Work out the finished part from the listing and answer in its coordinate system (mm). Face numbers are marked on the shaded views. A direction names the side the tool comes from. Coordinates: 2 decimals unless noted, no trailing zeros. Loops run counter-clockwise (first coordinate to the right, second up) from the corner with the lowest first, then second, coordinate; pieces in that order, holes last. Notation, with made-up numbers: (30.25, 65) - (61.25, 65) arc R8 ccw to (61.25, 75) - close; hole circle Ø3 at (27, 32). An arc over 180 degrees is marked (long way). Write each question's results on one line, items separated by ' | '. Start each with the question number.
1. Which of the six approach directions +Z, -Z, +X, -X, +Y, -Y give full straight-line access (tool end or side, diameter ignored) to the marked faces 1, 2 and 3?
2. Determine the mould class of the marked faces 4, 5, 6 and 7 for opening direction Z: released by +Z, released by -Z, zero draft, split by the parting line, or undercut.
3. A cutting plane is placed at C-C on z = 0. State how many separate pieces and enclosed holes the cut face has, then the cut area to 3 significant figures.
4. A cutting plane is placed at A-A on x = 16. Determine the outline of the cut face in (y, z), then the cut area to 3 significant figures.
5. Each of these flat-tipped pins is pushed along its axis until it touches: P1, Ø2.5, axis at x = -5.5, z = 1, coming from the -Y side; P2, Ø1, axis at x = 2, z = 0, coming from the +Y side; P3, Ø1.5, axis at y = 11.5, z = -0.5, coming from the -X side. Where does it stop, or does it pass through?
6. Find the intervals of material crossed by line 1 along Y through (x, z) = (16, 2.35); line 2 along Z through (x, y) = (0, 7.8); line 3 along X through (y, z) = (10, 0.65), in increasing order. Write a range as [from, to].
7. A cutting plane is placed at D-D on x = -10. Determine the outline of the cut face in (y, z).
8. A cutting plane is placed at B-B on y = -2. Determine the outline of the cut face in (x, z), then the cut area to 3 significant figures.
from build123d import *

# Parameters (mm, degrees)
F0_R     = 1.5
F0_W     = 2
F0_H     = 5
F1_DEPTH = 2.5
F2_R     = 1.25
F2_R_2   = 1
F3_DEPTH = 9.001
F4_W     = 10
F4_H     = 3
F5_DEPTH = 19.001
F6_R     = 1
F7_DEPTH = 4
F8_R     = 1
F9_DEPTH = 18.001


with BuildPart() as f1:
    # F0 (on Top) → F1 (new body, symmetric)
    with BuildSketch(Plane.XY):
        Polygon((23, -5), (23, 5), (13, 5), (13, 9), (6, 9), (4, 9), (-4, 9), (-6, 9), (-12, 9), (-12, 5), (7.5, 5), (7.5, -5), align=None)
        with Locations((16, 0)):
            Circle(F0_R, mode=Mode.SUBTRACT)
        with Locations((5, 11.5)):
            Rectangle(F0_W, F0_H)
        with Locations((-5, 11.5)):
            Rectangle(F0_W, F0_H)
    extrude(amount=F1_DEPTH, both=True)

    # F2 (on face) → F3 (cut, through all)
    with BuildSketch(Plane.XZ.offset(-5)):
        Circle(F2_R)
        with Locations((-10, 0)):
            Circle(F2_R_2)
    extrude(amount=-F3_DEPTH, mode=Mode.SUBTRACT)

    # F4 (on face) → F5 (cut, through all)
    with BuildSketch(Plane.XZ.offset(5)):
        with Locations((18, 0)):
            Rectangle(F4_W, F4_H)
    extrude(amount=-F5_DEPTH, mode=Mode.SUBTRACT)

    # F6 (on face) → F7 (cut)
    with BuildSketch(Plane.XZ.offset(5)):
        with Locations((10, 0)):
            Circle(F6_R)
    extrude(amount=-F7_DEPTH, mode=Mode.SUBTRACT)

    # F8 (on face) → F9 (cut, through all)
    with BuildSketch(Plane.YZ.offset(6)):
        with Locations((11.5, 0)):
            Circle(F8_R)
    extrude(amount=-F9_DEPTH, mode=Mode.SUBTRACT)


solid = f1.part
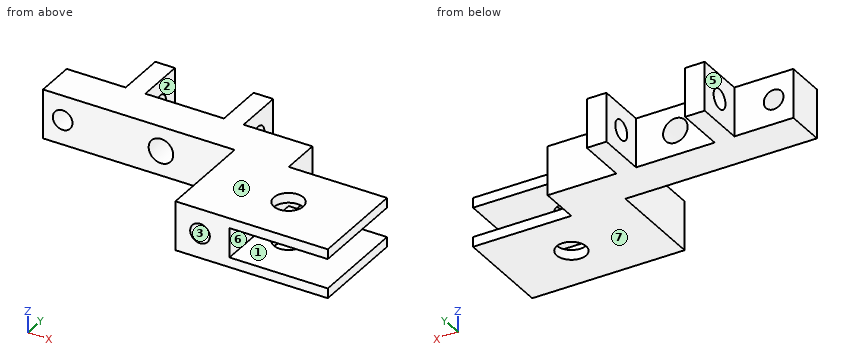
Values:
1) face 1: +X, +Y, -Y | face 2: +Z, -Z, +Y | face 3: -Y
2) face 4: released by +Z | face 5: zero draft | face 6: undercut | face 7: released by -Z
3) separate pieces: 5 | enclosed holes: 0 | area: 141 mm^2
4) outline: (-5, -2.5) - (-1.5, -2.5) - (-1.5, -1.5) - (-5, -1.5) - close; (-5, 1.5) - (-1.5, 1.5) - (-1.5, 2.5) - (-5, 2.5) - close; (1.5, -2.5) - (5, -2.5) - (5, -1.5) - (1.5, -1.5) - close; (1.5, 1.5) - (5, 1.5) - (5, 2.5) - (1.5, 2.5) - close | area: 14.0 mm^2
5) P1: y = 5 | P2: y = 9 | P3: x = -6
6) line 1: [-5, -1.5], [1.5, 5] | line 2: [-2.5, -1.25], [1.25, 2.5] | line 3: [-6, -4], [4, 6]
7) outline: (5, -2.5) - (9, -2.5) - (9, -1) - (5, -1) - close; (5, 1) - (9, 1) - (9, 2.5) - (5, 2.5) - close
8) outline: (7.5, -2.5) - (23, -2.5) - (23, -1.5) - (13, -1.5) - (13, 1.5) - (23, 1.5) - (23, 2.5) - (7.5, 2.5) - close; hole circle Ø2 at (10, 0) | area: 44.4 mm^2
